Build history of the part. All positions in model axes, mm. Face numbers are marked on the shaded views. Round coordinates to 2 decimals unless told otherwise and drop trailing zeros. Use one line per item in the form item = value. Start each with the question number.
```python
from build123d import *

# Parameters (mm, degrees)
F1_R     = 0.05
F2_DEPTH = 6.6
F3_DEPTH = 0.05
F4_R     = 6


# Not quite as in the source:
# - a feature names something its author has since deleted; it is built from what else it names


with BuildPart() as f2:
    # F1 (on Top) → F2 (new body, symmetric)
    with BuildSketch(Plane.XY):
        with BuildLine():
            ThreePointArc((-22.0188386326, -14.3586602491), (-17.4326418198, -12.0110708593), (-15.5892822956, -7.2))
            ThreePointArc((-15.5892822956, -7.2), (-17.6078830939, -2.2006898163), (-22.5318107159, -0.004605057))
            ThreePointArc((-22.5318107159, -0.004605057), (-29.9846889937, -7.4571428571), (-22.0188386326, -14.3586602491))
        make_face()
        with Locations((-22.7892822956, -7.2)):
            Circle(F1_R, mode=Mode.SUBTRACT)
        with BuildLine():
            ThreePointArc((-22.5318107159, -0.004605057), (-17.6078830939, -2.2006898163), (-15.5892822956, -7.2))
            ThreePointArc((-15.5892822956, -7.2), (-17.4326418198, -12.0110708593), (-22.0188386326, -14.3586602491))
            Line((-22.0188386326, -14.3586602491), (-5.3579636142, -12.5655502076))
            ThreePointArc((-5.3579636142, -12.5655502076), (-11.9961722484, -6.8142857143), (-5.7854403503, -0.6038375475))
            Line((-5.7854403503, -0.6038375475), (-22.5318107159, -0.004605057))
        make_face()
        with BuildLine():
            ThreePointArc((0, -6.6), (-1.682167332, -2.4339081802), (-5.7854403503, -0.6038375475))
            ThreePointArc((-5.7854403503, -0.6038375475), (-11.9961722484, -6.8142857143), (-5.3579636142, -12.5655502076))
            ThreePointArc((-5.3579636142, -12.5655502076), (-1.5361329369, -10.6092257161), (0, -6.6))
        make_face()
        with Locations((-6, -6.6)):
            Circle(F1_R, mode=Mode.SUBTRACT)
        with Locations((-22.7892822956, -7.2)):
            Circle(F1_R)
        with Locations((-6, -6.6)):
            Circle(F1_R)
    extrude(amount=F2_DEPTH, both=True)

    # F1 (on Top) → F3 (cut, symmetric)
    with BuildSketch(Plane.XY):
        with Locations((-22.7892822956, -7.2)):
            Circle(F1_R)
        with Locations((-6, -6.6)):
            Circle(F1_R)
    extrude(amount=F3_DEPTH, both=True, mode=Mode.SUBTRACT)

    # F4
    f4_edges = [f2.edges().sort_by_distance(p)[0] for p in [
        (-29.984689, -7.457143, 6.6),
        (-13.688401, -13.462105, 6.6),
        (-0.003828, -6.385714, 6.6),
        (-14.158626, -0.304221, 6.6),
        (-29.984689, -7.457143, -6.6),
        (-13.688401, -13.462105, -6.6),
        (-0.003828, -6.385714, -6.6),
        (-14.158626, -0.304221, -6.6),
    ]]
    fillet(f4_edges, radius=F4_R)


solid = f2.part
```
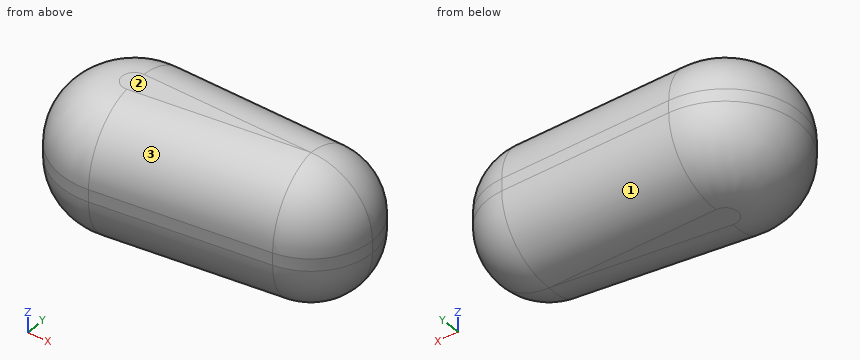
Q1. Pull direction Y, two halves, no side cores. Call the marked faces 1, 2 and 3: pulls with the +Y half, pulls with the -Y half, needs draft (parallel to the pull), parting line crosses it, or undercut.
Q2. Drop flat-ended pins along their axis: P1, Ø1, axis at x = -22.5, z = 4.5, coming from the -Y side; P2, Ø3, axis at x = -8, y = -9, coming from the +Z side; P3, Ø1.5, axis at y = -10.5, z = 2, coming from the +X side. Give the stop position or say it passes through.
Q3. Wall check: probe 1 along Y at (x, z) = (-15.5, -6); probe 2 along Z at (x, y) = (-24, -13.5); probe 3 along Z at (x, y) = (-16.5, -2). Give the ranges that are in metal, low to high.
Filled in:
q1.face_1 = pulls with the +Y half
q1.face_2 = needs draft
q1.face_3 = pulls with the -Y half
q2.P1 = -13.34
q2.P2 = 6.56
q2.P3 = -1.05
q3.probe_1 = -10.25 to -3.64
q3.probe_2 = -3.57 to 3.57
q3.probe_3 = -4.86 to 4.86
